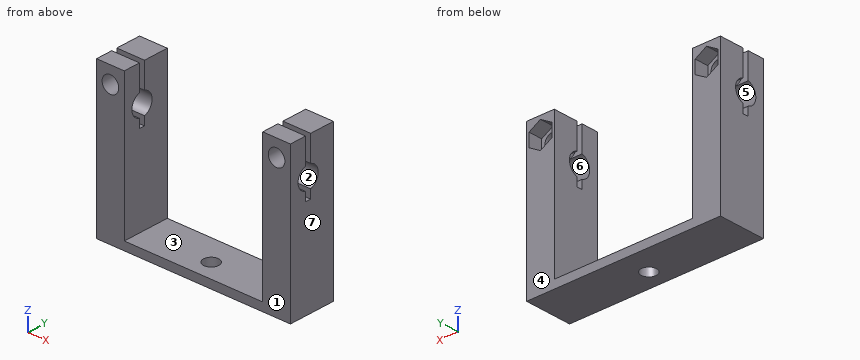
```python
from build123d import *

# Parameters (mm, degrees)
PAD_DEPTH       = 7
PAD_DEPTH_BACK  = 10
SKETCH003_R     = 4
POCKET_DEPTH    = 35.001
SKETCH004_R     = 3
POCKET001_DEPTH = 17.001
POCKET003_DEPTH = 5
SKETCH007_W     = 2
SKETCH007_H     = 20
POCKET004_DEPTH = 35.001
SKETCH008_R     = 2.75
POCKET005_DEPTH = 54.751


with BuildPart() as part:
    # Sketch → Pad (new body, two sides)
    with BuildSketch(Plane.XZ) as pad_sk:
        Polygon((0, 0), (0, 3), (25, 3), (25, 54.75), (35, 54.75), (35, 0), align=None)
    extrude(amount=PAD_DEPTH)
    extrude(pad_sk.sketch, amount=-PAD_DEPTH_BACK)

    # Sketch003 → Pocket (cut, through all)
    with BuildSketch(Plane.YZ):
        with Locations((0, 41.75)):
            Circle(SKETCH003_R)
    extrude(amount=POCKET_DEPTH, mode=Mode.SUBTRACT)

    # Sketch004 (on Face5 of Pocket) → Pocket001 (cut, through all)
    with BuildSketch(Plane.XZ.offset(7)):
        with Locations((30, 48.75)):
            Circle(SKETCH004_R)
    extrude(amount=-POCKET001_DEPTH, mode=Mode.SUBTRACT)

    # Sketch006 → Pocket003 (cut)
    with BuildSketch(Plane(origin=(0, 10, 0), x_dir=(1, 0, 0), z_dir=(0, 1, 0))):
        Polygon((30, -44), (25.886379, -46.375), (25.886379, -51.125), (30, -53.5), (34.113621, -51.125), (34.113621, -46.375), align=None)
    extrude(amount=-POCKET003_DEPTH, mode=Mode.SUBTRACT)

    # Sketch007 → Pocket004 (cut, through all)
    with BuildSketch(Plane.YZ):
        with Locations((0, 44.75)):
            Rectangle(SKETCH007_W, SKETCH007_H)
    extrude(amount=POCKET004_DEPTH, mode=Mode.SUBTRACT)

    # Mirrored: part across YZ


with BuildPart() as part_1:
    add(part.part)
    add(part.part.mirror(Plane.YZ))

    # Sketch008 → Pocket005 (cut, through all)
    with BuildSketch(Plane.XY):
        Circle(SKETCH008_R)
    extrude(amount=POCKET005_DEPTH, mode=Mode.SUBTRACT)


solid = part_1.part
```
Can you work these out from the model? Positions are in its coordinate system, mm. Face numbers are marked on the shaded views. A direction names the side the tool comes from. Give positions to 0.01 mm unless a question says otherwise; leave off trailing zeros. Loops run counter-clockwise (first coordinate to the right, second up) from the corner with the lowest first, then second, coordinate; pieces in that order, holes last. Notation, with made-up numbers: M 47.5,-3 L 60.5,-3 A24 ccw 60.5,17 Z; hole C 73,42 d5. An arc over 180 degrees is marked long. Answer in a Markdown table with one row per item.
1. For pin 1 Ø5.5 at (x, z) = (-30, 48.75) entering from +Y; pin 2 Ø2.5 at (x, z) = (30, 51.5) entering from +Y, each with a flat end and sliding along its axis, tell me the tip position at first contact or that it passes through.
Taken from the geometry:
| item | result |
|---|---|
| pin 1 | passes through |
| pin 2 | stops at y = 5 |
2. Suppose I cut it at D-D on z = 43. Write out the boundary of the cut face in (x, y).
Taken from the geometry:
| item | result |
|---|---|
| outline | M -35,-7 L -25,-7 L -25,-3.8 L -35,-3.8 Z; M -35,3.8 L -25,3.8 L -25,10 L -35,10 Z; M 25,-7 L 35,-7 L 35,-3.8 L 25,-3.8 Z; M 25,3.8 L 35,3.8 L 35,10 L 25,10 Z |
3. Suppose I cut it at B-B on y = 0. Write out the boundary of the cut face in (x, z), plus the area to 4 significant figures.
Taken from the geometry:
| item | result |
|---|---|
| outline | M -35,0 L -2.75,0 L -2.75,3 L -25,3 L -25,34.75 L -35,34.75 Z; M 2.75,0 L 35,0 L 35,34.75 L 25,34.75 L 25,3 L 2.75,3 Z |
| area | 828.5 mm² |
4. Suppose I cut it at C-C on z = 33. Write out the boundary of the cut face in (x, y), plus the area to 3 significant figures.
Taken from the geometry:
| item | result |
|---|---|
| outline | M -35,-7 L -25,-7 L -25,10 L -35,10 Z; M 25,-7 L 35,-7 L 35,10 L 25,10 Z |
| area | 340 mm² |
5. If I drill on line 1 along X through (y, z) = (-5.5, 28.5); line 2 along Z through (x, y) = (-30, -4.2); line 3 along X through (y, z) = (0, 0.75), over which ranges is the centre line in solid material (lowest first)?
Taken from the geometry:
| item | result |
|---|---|
| line 1 | x = -35 to -25, 25 to 35 |
| line 2 | z = 0 to 45.75, 51.75 to 54.75 |
| line 3 | x = -35 to -2.75, 2.75 to 35 |
6. Suppose I cut it at A-A on x = 0. Write out the boundary of the cut face in (y, z), plus the area to 3 significant figures.
Taken from the geometry:
| item | result |
|---|---|
| outline | M -7,0 L -2.75,0 L -2.75,3 L -7,3 Z; M 2.75,0 L 10,0 L 10,3 L 2.75,3 Z |
| area | 34.5 mm² |
7. Thinking about a two-plate mould opening in Y: for the marked faces 4, 5, 6 and 7, which applies, released by +Y, released by -Y, zero draft, split by the parting line, or undercut?
Taken from the geometry:
| item | result |
|---|---|
| face 4 | released by +Y |
| face 5 | undercut |
| face 6 | undercut |
| face 7 | zero draft |
8. Which directions (+Z, -Z, +X, -X, +Y, -Y) give clear straight access to the entire face, cutting with the end or side of a thin tool? Please do the marked faces 1, 2 and 3.
Taken from the geometry:
| item | result |
|---|---|
| face 1 | +Z, -Z, +X, -X, -Y |
| face 2 | +X, -X |
| face 3 | +Z, +Y, -Y |
